from build123d import *

# Parameters (mm, degrees)
CROQUIS1_W              = 28
CROQUIS1_H              = 28
CROQUIS1_W_2            = 20.4
CROQUIS1_H_2            = 20.4
SALIENTE_EXTRUIR1_DEPTH = 30.3
CROQUIS2_W              = 34
CROQUIS2_H              = 34
SALIENTE_EXTRUIR2_DEPTH = 31.5
CROQUIS3_R              = 12.625
CORTAR_EXTRUIR1_DEPTH   = 63
CROQUIS4_W              = 34
CROQUIS4_H              = 34
SALIENTE_EXTRUIR3_DEPTH = 2
CORTAR_EXTRUIR2_REACH   = 67
CROQUIS5_R              = 3.75
CORTAR_EXTRUIR3_REACH   = 36
CROQUIS6_W              = 15
CROQUIS6_H              = 11
CROQUIS7_W              = 34
CROQUIS7_H              = 34
CROQUIS7_W_2            = 31
CROQUIS7_H_2            = 31
CORTAR_EXTRUIR4_DEPTH   = 6
CROQUIS8_R              = 2
CORTAR_EXTRUIR7_DEPTH   = 40
CROQUIS10_R             = 4
CORTAR_EXTRUIR8_DEPTH   = 25.5
SALIENTE_EXTRUIR4_DEPTH = 4


with BuildPart() as part:
    # Croquis1 → Saliente-Extruir1 (new body)
    with BuildSketch(Plane(origin=(0, 0, 0), x_dir=(0, 0, -1), z_dir=(1, 0, 0))):
        Rectangle(CROQUIS1_W, CROQUIS1_H)
        Rectangle(CROQUIS1_W_2, CROQUIS1_H_2, mode=Mode.SUBTRACT)
    extrude(amount=SALIENTE_EXTRUIR1_DEPTH)

    # Croquis2 → Saliente-Extruir2 (add, symmetric)
    with BuildSketch(Plane(origin=(0, 0, 0), x_dir=(1, 0, 0), z_dir=(0, 1, 0))):
        with Locations((47.3, 0)):
            Rectangle(CROQUIS2_W, CROQUIS2_H)
    extrude(amount=SALIENTE_EXTRUIR2_DEPTH, both=True)

    # Croquis3 → Cortar-Extruir1 (cut)
    with BuildSketch(Plane.XZ.offset(31.5)):
        with Locations((47.3, 0)):
            Circle(CROQUIS3_R)
    extrude(amount=-CORTAR_EXTRUIR1_DEPTH, mode=Mode.SUBTRACT)

    # Croquis4 → Saliente-Extruir3 (add)
    with BuildSketch(Plane(origin=(0, 31.5, 0), x_dir=(1, 0, 0), z_dir=(0, 1, 0))):
        with Locations((47.3, 0)):
            Rectangle(CROQUIS4_W, CROQUIS4_H)
    extrude(amount=SALIENTE_EXTRUIR3_DEPTH)

    # Croquis5 → Cortar-Extruir2 (cut, up to next)
    with BuildSketch(Plane(origin=(0, 33.5, 0), x_dir=(1, 0, 0), z_dir=(0, 1, 0)), mode=Mode.PRIVATE) as cortar_extruir2_sk1:
        with Locations((47.3, 0)):
            Circle(CROQUIS5_R)
    cortar_extruir2_tool1 = extrude(cortar_extruir2_sk1.sketch, amount=-CORTAR_EXTRUIR2_REACH, mode=Mode.PRIVATE) & part.part
    add(cortar_extruir2_tool1.solids().sort_by_distance((47.3, 33.5, 0))[0], mode=Mode.SUBTRACT)

    # Croquis6 → Cortar-Extruir3 (cut, up to next)
    with BuildSketch(Plane.ZY.offset(-30.3), mode=Mode.PRIVATE) as cortar_extruir3_sk1:
        with Locations((0, -26)):
            Rectangle(CROQUIS6_W, CROQUIS6_H)
    cortar_extruir3_tool1 = extrude(cortar_extruir3_sk1.sketch, amount=-CORTAR_EXTRUIR3_REACH, mode=Mode.PRIVATE) & part.part
    add(cortar_extruir3_tool1.solids().sort_by_distance((30.3, -26, 0))[0], mode=Mode.SUBTRACT)

    # Croquis7 → Cortar-Extruir4 (cut)
    with BuildSketch(Plane.XZ.offset(31.5)):
        with Locations((47.3, 0)):
            Rectangle(CROQUIS7_W, CROQUIS7_H)
        with Locations((47.3, 0)):
            Rectangle(CROQUIS7_W_2, CROQUIS7_H_2, mode=Mode.SUBTRACT)
    extrude(amount=-CORTAR_EXTRUIR4_DEPTH, mode=Mode.SUBTRACT)

    # Croquis8 → Cortar-Extruir7 (cut)
    with BuildSketch(Plane.XY.offset(15.5)):
        with Locations((47.3, -28.5)):
            Circle(CROQUIS8_R)
    extrude(amount=-CORTAR_EXTRUIR7_DEPTH, mode=Mode.SUBTRACT)

    # Croquis10 → Cortar-Extruir8 (cut)
    with BuildSketch(Plane(origin=(0, 14, 0), x_dir=(1, 0, 0), z_dir=(0, 1, 0))):
        with Locations((15, 0)):
            Circle(CROQUIS10_R)
    extrude(amount=-CORTAR_EXTRUIR8_DEPTH, mode=Mode.SUBTRACT)

    # Croquis12 → Saliente-Extruir4 (add)
    with BuildSketch(Plane.ZY):
        Polygon((-8, 10.2), (-8, 14), (-14, 14), (-14, 8), (-10.2, 8), (-10.2, 10.2), align=None)
        Polygon((14, 10.2), (14, 14), (8, 14), (8, 10.2), (10.2, 10.2), (10.2, 8), (14, 8), align=None)
        Polygon((14, -14), (14, -8), (10.2, -8), (10.2, -10.2), (8, -10.2), (8, -14), align=None)
        Polygon((-10.2, -8), (-14, -8), (-14, -14), (-8, -14), (-8, -10.2), (-10.2, -10.2), align=None)
    extrude(amount=SALIENTE_EXTRUIR4_DEPTH)


solid = part.part
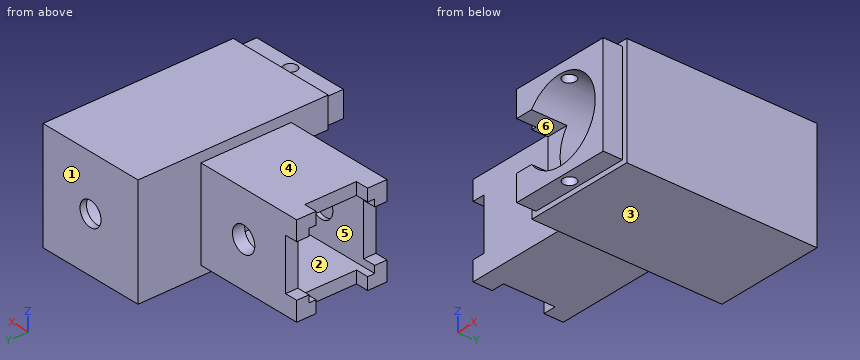
Source: CAD feature listing. Evaluate the final solid. Frame: model axes, mm. Face numbers are marked on the shaded views. A direction names the side the tool comes from. Coordinates: 2 decimals unless noted, no trailing zeros. Loops run counter-clockwise (first coordinate to the right, second up) from the corner with the lowest first, then second, coordinate; pieces in that order, holes last. Notation, with made-up numbers: (9.5, 66) - (39.5, 66) arc R30 cw to (39.5, 92) - close; hole circle Ø2 at (54.25, 74). An arc over 180 degrees is marked (long way). One line per item, written item: value. Start each with the question number.
1. Mould query, pull axis Y, two halves, no side actions, for the marked faces 1, 2 and 3. Classes: pulls with the +Y half, pulls with the -Y half, needs draft (parallel to the pull), parting line crosses it, or undercut.
2. Section C-C (x = 27.5). Return the cut outline in (y, z).
3. Contact query for flat-ended pins moving along their axis: P1, Ø1.5, axis at x = 4.5, y = -10, coming from the +Z side; P2, Ø4, axis at x = 4.5, y = -10.5, coming from the -Z side; P3, Ø3, axis at y = -0.5, z = 13, coming from the -X side. Output: stop coordinate, or through.
4. Ray query, L1, parallel to X at y = 11, z = 0 (3 decimals); L2, parallel to Z at x = 15, y = 11; L3, parallel to Z at x = 15, y = -10. Return the intervals inside material, ascending.
5. Set-up query: the marked faces 4, 5 and 6. Return all of +Z, -Z, +X, -X, +Y, -Y with unobstructed straight access to the full face (end or side cutting, diameter ignored); none if empty.
6. Section A-A (z = 0). State how many separate pieces and enclosed holes the cut face has, and give its area (3 significant figures).
7. Section B-B (x = 47.3). Return the cut outline in (y, z) (3 decimals).
8. Section D-D (y = -17). Return the cut outline in (x, z) (3 decimals).
Verdict:
1. face 1: pulls with the +Y half
1. face 2: undercut
1. face 3: needs draft
2. outline: (-14, -14) - (14, -14) - (14, 14) - (-14, 14) - close; hole (-10.2, -10.2) - (10.2, -10.2) - (10.2, 10.2) - (-10.2, 10.2) - close
3. P1: stops at z = 14
3. P2: stops at z = -14
3. P3: stops at x = 0
4. L1: x = 0 to 11, 19 to 34.675, 59.925 to 64.3
4. L2: z = -14 to -4, 4 to 14
4. L3: z = -14 to -10.2, 10.2 to 14
5. face 4: +Z, -X, +Y, -Y
5. face 5: -X
5. face 6: -X, -Y
6. separate pieces: 3
6. enclosed holes: 0
6. area: 737 mm2
7. outline: (-31.5, -15.5) - (-30.5, -15.5) - (-30.5, -12.625) - (-31.5, -12.625) - close; (-31.5, 12.625) - (-30.5, 12.625) - (-30.5, 15.5) - (-31.5, 15.5) - close; (-26.5, -15.5) - (-25.5, -15.5) - (-25.5, -17) - (33.5, -17) - (33.5, -3.75) - (31.5, -3.75) - (31.5, -12.625) - (-26.5, -12.625) - close; (-26.5, 12.625) - (31.5, 12.625) - (31.5, 3.75) - (33.5, 3.75) - (33.5, 17) - (-25.5, 17) - (-25.5, 15.5) - (-26.5, 15.5) - close
8. outline: (30.3, -17) - (64.3, -17) - (64.3, 17) - (30.3, 17) - close; hole circle Ø25.25 at (47.3, 0)
